Check sheet for the drawn part. Datum: minimum x, y, z corner. Units: mm. A direction names the side the tool comes from. Coordinates: 2 decimals unless noted, no trailing zeros. Order: outer loops, then holes, each group sorted by start corner. A loop starts at its lowest first (then second) coordinate and runs counter-clockwise, first axis right, second up. Notation, with made-up numbers: (32.25, -33) -> (43.25, -33) arc R19 cw to (43.25, -11) -> close; hole circle Ø4 at (-7.5, -35.75). An arc over 180 degrees is marked (long way). Answer as CSV lines item,"result".
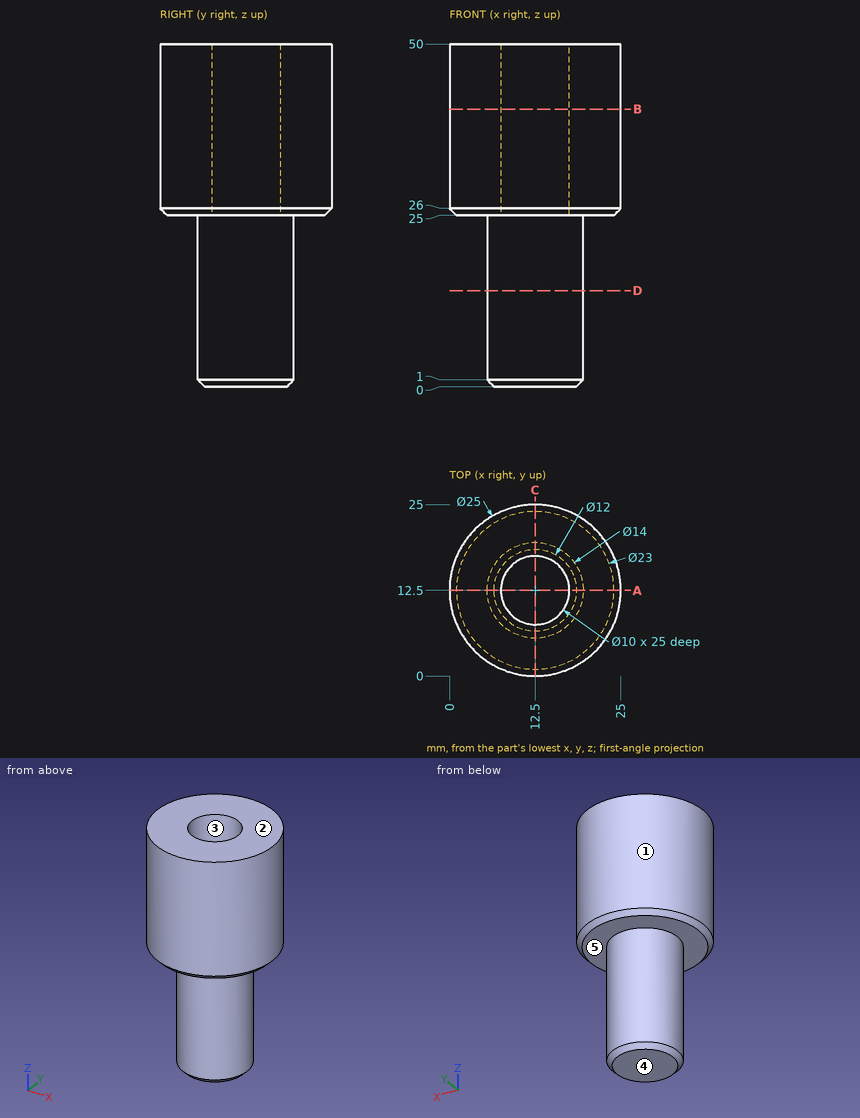
Item 1: Section check A-A, the plane y = 12.5. Record the boundary of the cut face in (x, z), plus the area to 3 significant figures.
Answer list:
outline,"(0, 26) -> (1, 25) -> (5.5, 25) -> (5.5, 1) -> (6.5, 0) -> (18.5, 0) -> (19.5, 1) -> (19.5, 25) -> (24, 25) -> (25, 26) -> (25, 50) -> (17.5, 50) -> (17.5, 25) -> (7.5, 25) -> (7.5, 50) -> (0, 50) -> close"
area,"723 mm2"
Item 2: Release check for a two-part mould opening along Y. For the marked faces 1, 2 and 3 record: +Y half, -Y half, draft (parallel to the pull), parting line (faces both ways), or undercut.
Answer list:
face 1,"parting line"
face 2,"draft"
face 3,"undercut"
Item 3: Tool access check on the marked faces 4 and 5. Record the directions out of +Z, -Z, +X, -X, +Y, -Y that give a thin tool (end or side, any length) a straight path to the whole face; none if there is none.
Answer list:
face 4,"-Z, +X, -X, +Y, -Y"
face 5,"-Z"
Item 4: Thickness scan on line 1 (Y direction, x = 12.5, z = 40.25); line 2 (Z direction, x = 12.25, y = 2.25); line 3 (Y direction, x = 11, z = 47). Record the ranges inside material, lowest first.
Answer list:
line 1,"0 to 7.5, 17.5 to 25"
line 2,"25 to 50"
line 3,"0.09 to 7.73, 17.27 to 24.91"
Item 5: Depth check by flat-ended pin: pin 1 Ø1.5 at (x, z) = (18, 36.5) entering from +Y; pin 2 Ø2 at (y, z) = (7.5, 19.5) entering from +X; pin 3 Ø3 at (x, y) = (8.5, 3.5) entering from -Z. Enter the tip coordinate at first touch or a pass-through.
Answer list:
pin 1,"y = 24.06"
pin 2,"x = 18.24"
pin 3,"z = 25"
Item 6: Section check B-B, the plane z = 40.5. Record the boundary of the cut face in (x, y).
Answer list:
outline,"circle Ø25 at (12.5, 12.5); hole circle Ø10 at (12.5, 12.5)"
Item 7: Section check D-D, the plane z = 14. Record the boundary of the cut face in (x, y), plus the area to 3 significant figures.
Answer list:
outline,"circle Ø14 at (12.5, 12.5)"
area,"154 mm2"
